Read the model definition and answer for the solid it produces. Units are mm, in the model's axes. Face numbers are marked on the shaded views. A direction names the side the tool comes from. Round coordinates to 2 decimals unless told otherwise and drop trailing zeros. Order: outer loops, then holes, each group sorted by start corner. A loop starts at its lowest first (then second) coordinate and runs counter-clockwise, first axis right, second up. Notation, with made-up numbers: (54, 5.25) - (109, 5.25) arc R8 ccw to (109, 16.25) - close; hole circle Ø4 at (64.25, -2.5). An arc over 180 degrees is marked (long way). Answer as a JSON object with one key per item and string values. Group by question number.
Q1. A cutting plane is placed at B-B on x = 19.5. Determine the outline of the cut face in (y, z), and give its area (3 significant figures).
Q2. A cutting plane is placed at D-D on x = 16. Determine the outline of the cut face in (y, z) (3 decimals).
Q3. A cutting plane is placed at A-A on x = 14. Determine the outline of the cut face in (y, z) (3 decimals).
Q4. Given pin 1 Ø4 at (x, y) = (14, -0.5) entering from -Z; pin 2 Ø1.9 at (x, y) = (15, 1) entering from +Z; pin 3 Ø7 at (x, y) = (18.5, -11) entering from +Z; pin 4 Ø4 at (x, z) = (14, -1.5) entering from +Y, each flat-ended and moving along its own axis, determine where each tip first touches the part or whether it passes through.
Q5. A tool of negligible diameter and unlimited length cuts with its end or side. For the marked faces 5, 6, 7 and 8, from which of +Z, -Z, +X, -X, +Y, -Y can it reach the whole face along a straight path? Write none if from no direction.
Q6. A cutting plane is placed at C-C on z = -2.25. Determine the outline of the cut face in (x, y) (3 decimals), and give its area (3 significant figures).
Q7. The mould has two halves that part along Y. Classify the marked faces 1, 2, 3 and 4: pulls with the +Y half, pulls with the -Y half, needs draft (parallel to the pull), parting line crosses it, or undercut.
Q8. Consider line 1 (Z direction, x = 19.5, y = -10.5); line 2 (Y direction, x = 22, z = -4.5); line 3 (X direction, y = 4, z = -8.25). Determine where each line is inside the solid, lowest interval first.
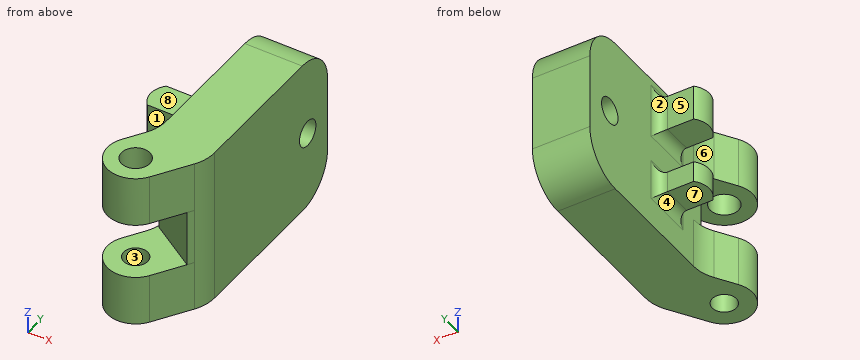
```python
from build123d import *

# Parameters (mm, degrees)
BOSS_EXTRUDE1_DEPTH = 6.35
BOSS_EXTRUDE2_DEPTH = 7.112
BOSS_EXTRUDE3_START = 6.35
BOSS_EXTRUDE3_DEPTH = 6.35
CUT_EXTRUDE1_REACH  = 37.909
SKETCH5_R           = 1.7907
CUT_EXTRUDE2_REACH  = 37.909
SKETCH6_R           = 1.524
SKETCH7_R           = 1.651
CUT_EXTRUDE3_DEPTH  = 24.282660099
SKETCH9_W           = 13
SKETCH9_H           = 3.81
BOSS_EXTRUDE4_DEPTH = 5.334
CUT_EXTRUDE4_DEPTH  = 34.50981373
SKETCH11_W          = 5.842
SKETCH11_H          = 8.036223638
CUT_EXTRUDE5_DEPTH  = 23.149777145
FILLET2_R           = 1.27
FILLET3_R           = 5.08
FILLET4_R           = 5.08


with BuildPart() as part:
    # Sketch2 → Boss-Extrude1 (new body)
    with BuildSketch(Plane.XY):
        with BuildLine():
            Line((21.644583215, -14.393094274), (25.301992713, -8.71448479))
            Line((25.301992713, -8.71448479), (25.301992713, 15.4724))
            Line((25.301992713, 15.4724), (18.047240712, 15.4724))
            Line((18.047240712, 15.4724), (18.047240712, -6.844010681))
            Line((18.047240712, -6.844010681), (15.665416785, -10.542105726))
            ThreePointArc((15.665416785, -10.542105726), (16.729505726, -15.457183215), (21.644583215, -14.393094274))
        make_face()
    extrude(amount=BOSS_EXTRUDE1_DEPTH)

    # Sketch3 → Boss-Extrude2 (add)
    with BuildSketch(Plane(origin=(0, 0, 0), x_dir=(-1, 0, 0), z_dir=(0, 0, -1))):
        Polygon((-18.047240712, -6.844010681), (-24.026407143, -10.694999229), (-25.301992713, -8.71448479), (-25.301992713, 15.4724), (-18.047240712, 15.4724), align=None)
    extrude(amount=BOSS_EXTRUDE2_DEPTH)

    # Sketch4 → Boss-Extrude3 (add)
    with BuildSketch(Plane(origin=(0, 0, -7.112), x_dir=(-1, 0, 0), z_dir=(0, 0, -1)).offset(BOSS_EXTRUDE3_START)):
        with BuildLine():
            Line((-25.301992713, 15.4724), (-25.301992713, -8.71448479))
            Line((-25.301992713, -8.71448479), (-21.644583215, -14.393094274))
            ThreePointArc((-21.644583215, -14.393094274), (-16.729505726, -15.457183215), (-15.665416785, -10.542105726))
            Line((-15.665416785, -10.542105726), (-18.047240712, -6.844010681))
            Line((-18.047240712, -6.844010681), (-18.047240712, 15.4724))
            Line((-18.047240712, 15.4724), (-25.301992713, 15.4724))
        make_face()
    extrude(amount=-BOSS_EXTRUDE3_DEPTH)

    # Sketch5 → Cut-Extrude1 (cut, up to next)
    with BuildSketch(Plane.XY.offset(6.35), mode=Mode.PRIVATE) as cut_extrude1_sk1:
        with Locations((18.655, -12.4676)):
            Circle(SKETCH5_R)
    cut_extrude1_tool1 = extrude(cut_extrude1_sk1.sketch, amount=-CUT_EXTRUDE1_REACH, mode=Mode.PRIVATE) & part.part
    add(cut_extrude1_tool1.solids().sort_by_distance((18.655, -12.4676, 6.35))[0], mode=Mode.SUBTRACT)

    # Sketch6 → Cut-Extrude2 (cut, up to next)
    with BuildSketch(Plane(origin=(0, 0, -13.462), x_dir=(-1, 0, 0), z_dir=(0, 0, -1)), mode=Mode.PRIVATE) as cut_extrude2_sk1:
        with Locations((-18.655, -12.4676)):
            Circle(SKETCH6_R)
    cut_extrude2_tool1 = extrude(cut_extrude2_sk1.sketch, amount=-CUT_EXTRUDE2_REACH, mode=Mode.PRIVATE) & part.part
    add(cut_extrude2_tool1.solids().sort_by_distance((18.655, -12.4676, -13.462))[0], mode=Mode.SUBTRACT)

    # Sketch7 → Cut-Extrude3 (cut, through all)
    with BuildSketch(Plane(origin=(25.301992713, 0, 0), x_dir=(0, 0, -1), z_dir=(1, 0, 0))):
        with Locations(Location((3.556, 11.47952, 0), (0, 0, 90))):
            Circle(SKETCH7_R)
    extrude(amount=-CUT_EXTRUDE3_DEPTH, mode=Mode.SUBTRACT)

    # Sketch9 → Boss-Extrude4 (add)
    with BuildSketch(Plane.ZY.offset(-18.047240712)):
        with Locations((-2.182, 0.00126)):
            Rectangle(SKETCH9_W, SKETCH9_H)
    extrude(amount=BOSS_EXTRUDE4_DEPTH)

    # Sketch10 → Cut-Extrude4 (cut, through all)
    with BuildSketch(Plane(origin=(0, 0, -8.682), x_dir=(-1, 0, 0), z_dir=(0, 0, -1))):
        with BuildLine():
            Line((-13.475240712, 1.90626), (-13.475240712, 3.862647324))
            Line((-13.475240712, 3.862647324), (-11.787992586, 3.862647324))
            Line((-11.787992586, 3.862647324), (-11.787992586, -3.9659176))
            Line((-11.787992586, -3.9659176), (-13.475240712, -3.9659176))
            Line((-13.475240712, -3.9659176), (-13.475240712, -1.90374))
            ThreePointArc((-13.475240712, -1.90374), (-12.713240712, 0.00126), (-13.475240712, 1.90626))
        make_face()
    extrude(amount=-CUT_EXTRUDE4_DEPTH, mode=Mode.SUBTRACT)

    # Sketch11 → Cut-Extrude5 (cut, through all)
    with BuildSketch(Plane.ZY.offset(-18.047240712)):
        with Locations((-3.094, 0.00126)):
            Rectangle(SKETCH11_W, SKETCH11_H)
    extrude(amount=CUT_EXTRUDE5_DEPTH, mode=Mode.SUBTRACT)

    # Fillet2
    fillet2_edges = [part.edges().sort_by_distance(p)[0] for p in [
        (18.047240712, -1.90374, 2.0725),
        (18.047240712, 1.90626, -7.3485),
        (18.047240712, 0.00126, -0.173),
        (18.047240712, 0.00126, -6.015),
        (18.047240712, 0.00126, 4.318),
        (18.047240712, 1.90626, 2.0725),
        (18.047240712, 0.00126, -8.682),
        (18.047240712, -1.90374, -7.3485),
    ]]
    fillet(fillet2_edges, radius=FILLET2_R)

    # Fillet3
    fillet3_edges = [part.edges().sort_by_distance(p)[0] for p in [
        (21.674616713, 15.4724, -13.462),
        (21.674616713, 15.4724, 6.35),
    ]]
    fillet(fillet3_edges, radius=FILLET3_R)

    # Fillet4
    fillet4_edges = [part.edges().sort_by_distance(p)[0] for p in [
        (25.301992713, -8.71448479, -3.556),
        (18.047240712, -6.844010681, 3.175),
        (18.047240712, -6.844010681, -10.287),
    ]]
    fillet(fillet4_edges, radius=FILLET4_R)


solid = part.part
```
Result set:
{
 "1": {"outline": "(-15.92, -13.46) - (-13.74, -13.46) - (-13.74, -7.11) - (-15.92, -7.11) - close; (-15.92, 0) - (-14.05, 0) - (-14.05, 6.35) - (-15.92, 6.35) - close; (-11.2, -13.46) - (10.39, -13.46) arc R5.08 ccw to (15.47, -8.38) - (15.47, 1.27) arc R5.08 ccw to (10.39, 6.35) - (-10.89, 6.35) - (-10.89, 0) - (-7.78, 0) - (-7.78, -7.11) - (-11.2, -7.11) - close; hole circle Ø3.3 at (11.48, -3.56)", "area": "508 mm²"},
 "2": {"outline": "(-14.833, -13.462) - (-10.023, -13.462) - (-10.023, -7.112) - (-14.833, -7.112) - close; (-14.833, 0) - (-10.023, 0) - (-10.023, 6.35) - (-14.833, 6.35) - close; (-1.904, -8.682) - (1.906, -8.682) - (1.906, -6.015) - (-1.904, -6.015) - close; (-1.904, -0.173) - (1.906, -0.173) - (1.906, 4.318) - (-1.904, 4.318) - close"},
 "3": {"outline": "(-1.904, -8.682) - (1.906, -8.682) - (1.906, -6.015) - (-1.904, -6.015) - close; (-1.904, -0.173) - (1.906, -0.173) - (1.906, 4.318) - (-1.904, 4.318) - close"},
 "4": {"pin 1": "stops at z = -8.68", "pin 2": "stops at z = 4.32", "pin 3": "stops at z = 6.35", "pin 4": "stops at y = 1.91"},
 "5": {"face 5": "+Z, -Z, -X, +Y", "face 6": "+Z, -Z, -X", "face 7": "-Z, -X, +Y", "face 8": "+Z, -X, +Y"},
 "6": {"outline": "(18.047, -6.844) - (24.026, -10.695) - (24.493, -9.971) arc R5.08 ccw to (25.302, -7.22) - (25.302, 10.469) - (18.047, 10.469) - close; (18.047, 12.49) - (25.302, 12.49) - (25.302, 15.472) - (18.047, 15.472) - close", "area": "162 mm²"},
 "7": {"face 1": "undercut", "face 2": "pulls with the +Y half", "face 3": "undercut", "face 4": "needs draft"},
 "8": {"line 1": "z = -13.46 to -7.11, 0 to 6.35", "line 2": "y = -9.39 to 10.13, 12.83 to 15.47", "line 3": "x = 18.05 to 25.3"}
}
